Can you work these out from the model? Positions are in its coordinate system, mm. A direction names the side the tool comes from. Coordinates: 2 decimals unless noted, no trailing zeros. Order: outer loops, then holes, each group sorted by start corner. A loop starts at its lowest first (then second) coordinate and runs counter-clockwise, first axis right, second up. Notation, with made-up numbers: (-24, 79.25) - (29, 79.25) arc R16 cw to (29, 85.25) - close; hole circle Ø8 at (34, 62.5). An arc over 180 degrees is marked (long way). Return JSON: item names as keys, results as strings. Group by question number.
1) Imagine slicing it at C-C (x = -12.25). Write out the boundary of the cut face in (y, z).
2) Imagine slicing it at B-B (y = 1.35). Write out the boundary of the cut face in (x, z).
3) Imagine slicing it at D-D (z = 7.5). Write out the boundary of the cut face in (x, y), and give its area (3 significant figures).
4) If we mould it in two halves opening along Z, with no side actions, what happens to faces 5 (the face through (-13.469, 1.676, -7.764)), 6 (the face through (-7, 2, -10.089)), 7 (the face through (-0.934, 3, 1))? For each: pulls with the +Z half, pulls with the -Z half, needs draft (parallel to the pull), parting line crosses it, or undercut.
5) For pin 1 Ø1.3 at (x, z) = (-3.93, -8.09) entering from -Y, with a flat end and sliding along its axis, tell me the tip position at first contact or that it passes through.
6) Which directions (+Z, -Z, +X, -X, +Y, -Y) give clear straight access to the entire face, cutting with the end or side of a thin tool? Please do faces 1 (the face through (-6.4, 3.1, 0.6)), 2 (the face through (-2, 1, -4)), 3 (the face through (-4, 2.6, 2.661)), 4 (the face through (-4, 0.5, 3.411)).
7) Imagine slicing it at A-A (z = 1.75). Write out the boundary of the cut face in (x, y), and give its area (3 significant figures).
8) If I drill on line 1 along Y through (x, z) = (-5.5, 6.5); line 2 along Z through (x, y) = (-3.25, 0.8); line 3 along Y through (x, z) = (-4.75, 9.5), over which ranges is the centre line in solid material (lowest first)?
```python
from build123d import *

# Parameters (mm, degrees)
SKETCH1_W                          = 21.5
SKETCH1_H                          = 21.5
BOSS_EXTRUDE1_DEPTH                = 3.1
SKETCH2_W                          = 5.5
SKETCH2_H                          = 1.1
CUT_EXTRUDE1_DEPTH                 = 27.219811656
SKETCH3_W                          = 21.5
SKETCH3_H                          = 21.5
SKETCH3_W_2                        = 5.5
SKETCH3_H_2                        = 5.5
BOSS_EXTRUDE2_DEPTH                = 0.3
SKETCH11_W                         = 4
SKETCH11_H                         = 4
CUT_EXTRUDE2_DEPTH                 = 19.85301637
TAP_DRILL_FOR_M2X0_4_TAP3_D        = 1.7
TAP_DRILL_FOR_M2_5X0_45_TAP1_D     = 2.15
TAP_DRILL_FOR_M2_5X0_45_TAP1_DEPTH = 1
CUT_EXTRUDE3_REACH                 = 20.905
SKETCH18_W                         = 5.5
SKETCH18_H                         = 5.5
FILLET3_R                          = 1
SKETCH21_W                         = 13.124555245
SKETCH21_H                         = 35.298127434
CUT_EXTRUDE8_DEPTH                 = 19.904661496
SKETCH22_W                         = 0.25
SKETCH22_H                         = 1.1
CUT_EXTRUDE9_DEPTH                 = 27.256970946


with BuildPart() as part:
    # Sketch1 → Boss-Extrude1 (new body)
    with BuildSketch(Plane(origin=(0, 0, 0), x_dir=(1, 0, 0), z_dir=(0, 1, 0))):
        with Locations((-3.933954619, -0.660858995)):
            Rectangle(SKETCH1_W, SKETCH1_H)
    extrude(amount=BOSS_EXTRUDE1_DEPTH)

    # Sketch2 → Cut-Extrude1 (cut, through all)
    with BuildSketch(Plane.XY.offset(11.410858995)):
        with Locations((-3.933954619, 1.55)):
            Rectangle(SKETCH2_W, SKETCH2_H)
    extrude(amount=-CUT_EXTRUDE1_DEPTH, mode=Mode.SUBTRACT)

    # Sketch3 → Boss-Extrude2 (add)
    with BuildSketch(Plane(origin=(0, 3.1, 0), x_dir=(1, 0, 0), z_dir=(0, 1, 0))):
        with Locations((-3.933954619, -0.660858995)):
            Rectangle(SKETCH3_W, SKETCH3_H)
        with Locations((-3.933954619, -0.660858995)):
            Rectangle(SKETCH3_W_2, SKETCH3_H_2, mode=Mode.SUBTRACT)
    extrude(amount=BOSS_EXTRUDE2_DEPTH)

    # Sketch11 → Cut-Extrude2 (cut, through all)
    with BuildSketch(Plane(origin=(0, 3.1, 0), x_dir=(1, 0, 0), z_dir=(0, 1, 0))):
        with Locations((-3.933954619, -0.660858995)):
            Rectangle(SKETCH11_W, SKETCH11_H)
    extrude(amount=-CUT_EXTRUDE2_DEPTH, mode=Mode.SUBTRACT)

    # Tap Drill for M2x0.4 Tap3 (through all)
    with Locations(Plane(origin=(0, 3.4, 0), x_dir=(1, 0, 0), z_dir=(0, 1, 0))):
        with Locations((-12.683954619, 8.089141005), (4.816045381, 8.089141005), (4.816045381, -9.410858995), (-12.683954619, -9.410858995), (-12.683954619, 3.709141005), (-12.683954619, -0.670858995), (-12.683954619, -5.050858995)):
            Hole(TAP_DRILL_FOR_M2X0_4_TAP3_D / 2)

    # Tap Drill for M2.5x0.45 Tap1
    with Locations(Plane(origin=(0, 0, 0), x_dir=(-1, 0, 0), z_dir=(0, -1, 0))):
        with Locations((3.933954619, 8.089141005), (3.933954619, -9.410858995), (3.933954619, 4.539141005), (3.933954619, -5.860858995)):
            Hole(TAP_DRILL_FOR_M2_5X0_45_TAP1_D / 2, depth=TAP_DRILL_FOR_M2_5X0_45_TAP1_DEPTH)

    # Sketch18 → Cut-Extrude3 (cut, up to next)
    with BuildSketch(Plane.XZ, mode=Mode.PRIVATE) as cut_extrude3_sk1:
        with Locations((-3.933954619, 0.660858995)):
            Rectangle(SKETCH18_W, SKETCH18_H)
    cut_extrude3_tool1 = extrude(cut_extrude3_sk1.sketch, amount=-CUT_EXTRUDE3_REACH, mode=Mode.PRIVATE) & part.part
    add(cut_extrude3_tool1.solids().sort_by_distance((-3.933955, 0, 0.660859))[0], mode=Mode.SUBTRACT)

    # Fillet3
    fillet3_edges = [part.edges().sort_by_distance(p)[0] for p in [
        (-14.683954619, 1.7, -10.089141005),
        (6.816045381, 1.7, -10.089141005),
        (6.816045381, 1.7, 11.410858995),
        (-14.683954619, 1.7, 11.410858995),
    ]]
    fillet(fillet3_edges, radius=FILLET3_R)

    # Sketch21 → Cut-Extrude8 (cut, through all)
    with BuildSketch(Plane(origin=(0, 3.4, 0), x_dir=(1, 0, 0), z_dir=(0, 1, 0))):
        with Locations((5.628323004, -1.911462044)):
            Rectangle(SKETCH21_W, SKETCH21_H)
    extrude(amount=-CUT_EXTRUDE8_DEPTH, mode=Mode.SUBTRACT)

    # Sketch22 → Cut-Extrude9 (cut, through all)
    with BuildSketch(Plane(origin=(0, 0, -10.089141005), x_dir=(-1, 0, 0), z_dir=(0, 0, -1))):
        with Locations((1.058954619, 1.55)):
            Rectangle(SKETCH22_W, SKETCH22_H)
    extrude(amount=-CUT_EXTRUDE9_DEPTH, mode=Mode.SUBTRACT)


solid = part.part
```
Calculated:
{
 "1": {"outline": "(0, -10.09) - (3.4, -10.09) - (3.4, -8.82) - (0, -8.82) - close; (0, -7.36) - (3.4, -7.36) - (3.4, -4.44) - (0, -4.44) - close; (0, -2.98) - (3.4, -2.98) - (3.4, -0.06) - (0, -0.06) - close; (0, 1.4) - (3.4, 1.4) - (3.4, 4.32) - (0, 4.32) - close; (0, 5.78) - (3.4, 5.78) - (3.4, 8.68) - (0, 8.68) - close; (0, 10.14) - (3.4, 10.14) - (3.4, 11.41) - (0, 11.41) - close"},
 "2": {"outline": "(-14.68, -9.09) arc R1 ccw to (-13.68, -10.09) - (-6.68, -10.09) - (-6.68, 11.41) - (-13.68, 11.41) arc R1 ccw to (-14.68, 10.41) - close; hole circle Ø1.7 at (-12.68, -8.09); hole circle Ø1.7 at (-12.68, -3.71); hole circle Ø1.7 at (-12.68, 0.67); hole circle Ø1.7 at (-12.68, 5.05); hole circle Ø1.7 at (-12.68, 9.41)"},
 "3": {"outline": "(-14.68, 0) - (-0.93, 0) - (-0.93, 1) - (-6.68, 1) - (-6.68, 2.1) - (-0.93, 2.1) - (-0.93, 3.4) - (-14.68, 3.4) - close", "area": "40.4 mm2"},
 "4": {"face 5": "undercut", "face 6": "pulls with the -Z half", "face 7": "needs draft"},
 "5": {"pin 1": "y = 2.1"},
 "6": {"face 1": "+Y", "face 2": "+Z, -Z, +X", "face 3": "+Y, -Y", "face 4": "-Y"},
 "7": {"outline": "(-14.68, 0) - (-6.68, 0) - (-6.68, 2.1) - (-5.93, 2.1) - (-5.93, 3.1) - (-6.68, 3.1) - (-6.68, 3.4) - (-14.68, 3.4) - close; (-1.93, 2.1) - (-0.93, 2.1) - (-0.93, 3.4) - (-1.18, 3.4) - (-1.18, 3.1) - (-1.93, 3.1) - close; (-1.18, 0) - (-0.93, 0) - (-0.93, 1) - (-1.18, 1) - close", "area": "29.3 mm2"},
 "8": {"line 1": "0 to 1, 2.1 to 3.4", "line 2": "-10.09 to -8.92, -7.26 to -5.37, -3.71 to -2.09, 3.41 to 5.03, 6.69 to 8.58, 10.24 to 11.41", "line 3": "2.1 to 3.4"}
}
